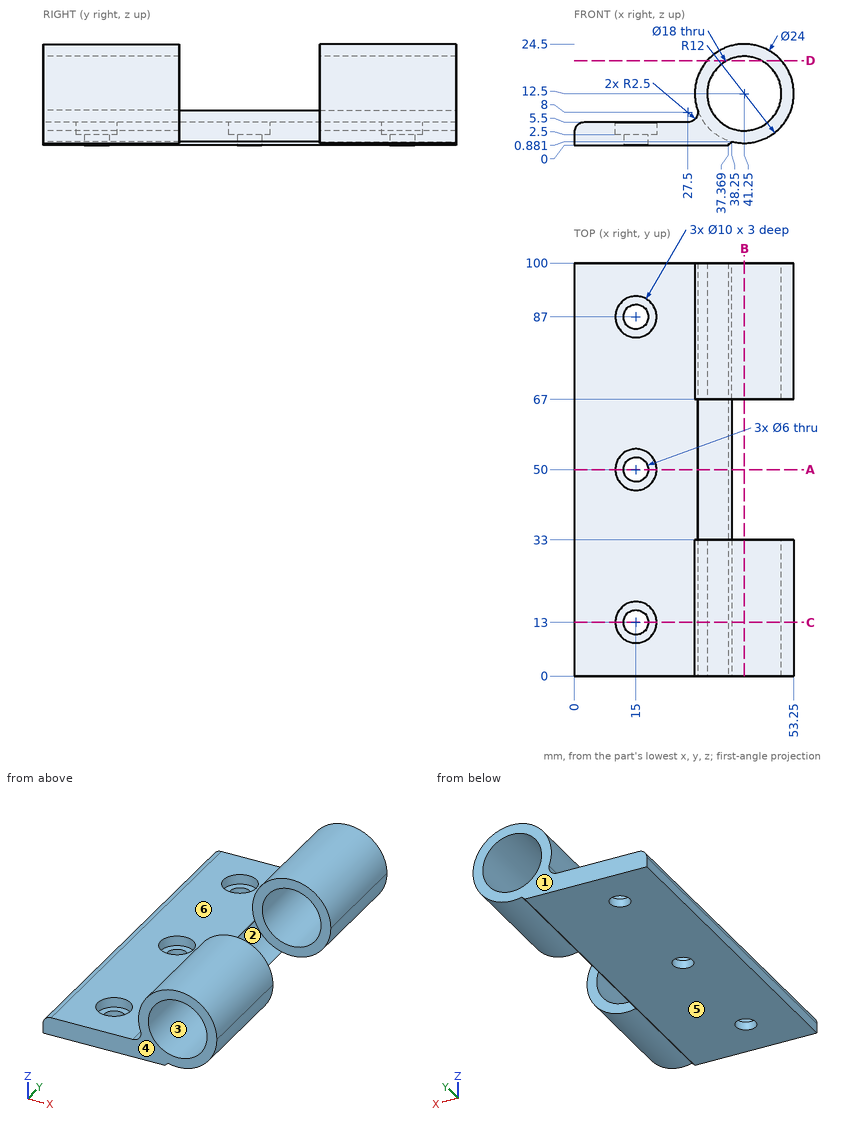
Geometry check sheet. Reference: drawing and pictorial views, mm from the part's lowest x, y, z. A direction names the side the tool comes from. Give positions to 0.01 mm unless a question says otherwise; leave off trailing zeros. Loops run counter-clockwise (first coordinate to the right, second up) from the corner with the lowest first, then second, coordinate; pieces in that order, holes last. Notation, with made-up numbers: (72, 53.25) - (102, 53.25) arc R33 cw to (102, 83.25) - close; hole circle Ø1 at (-5.5, -19.5). An arc over 180 degrees is marked (long way). Use CSV: the item, a comma, the result in double quotes. Start each with the question number.
Q1. Access from +Z, -Z, +X, -X, +Y, -Y to the whole of each face (thin tool, end or side, straight path). Record for the marked faces 1 and 2.
Q2. Go/stop test with flat-tipped pins: pin 1 Ø8 at (y, z) = (89, 4) entering from +X; pin 2 Ø1 at (x, y) = (8, 30) entering from -Z; pin 3 Ø9.5 at (x, y) = (15, 87) entering from +Z; pin 4 Ø11 at (x, y) = (13, 48) entering from +Z. Record where each tip stops, or that it passes through.
Q3. Section check A-A, the plane y = 50. Record the cut outline in (x, z), and give its area (3 significant figures).
Q4. Release check for a two-part mould opening along Z. For the marked faces 3, 4, 5 and 6 record: +Z half, -Z half, draft (parallel to the pull), parting line (faces both ways), or undercut.
Q5. Section check C-C, the plane y = 13. Record the cut outline in (x, z), and give its area (3 significant figures).
Q6. Section check B-B, the plane x = 41.25. Record the cut outline in (y, z).
Q7. Scan lines: probe 1 along Y at (x, z) = (15, 1.65); probe 2 along Z at (x, y) = (41.25, 19.5); probe 3 along Y at (x, z) = (34, 3). Record each from-to range of solid material in increasing order. Write a range as from..to.
Q8. Section check D-D, the plane z = 20.5. Record the cut outline in (x, y).
Findings below:
1,face 1,"+Z, -Z, +X, -X, +Y"
1,face 2,"+Z, +X"
2,pin 1,"stops at x = 52.37"
2,pin 2,"stops at z = 0"
2,pin 3,"stops at z = 2.5"
2,pin 4,"stops at z = 5.5"
3,outline,"(0, 0) - (12, 0) - (12, 2.5) - (10, 2.5) - (10, 5.5) - (2.5, 5.5) arc R2.5 ccw to (0, 3) - close; (18, 0) - (37.37, 0) - (38.25, 0.88) arc R12 cw to (29.96, 8.42) arc R2.5 cw to (27.5, 5.5) - (20, 5.5) - (20, 2.5) - (18, 2.5) - close"
3,area,"147 mm^2"
4,face 3,"undercut"
4,face 4,"draft"
4,face 5,"-Z half"
4,face 6,"+Z half"
5,outline,"(0, 0) - (12, 0) - (12, 2.5) - (10, 2.5) - (10, 5.5) - (2.5, 5.5) arc R2.5 ccw to (0, 3) - close; (18, 0) - (37.37, 0) - (38.25, 0.88) arc R12 ccw (long way) to (29.96, 8.42) arc R2.5 cw to (27.5, 5.5) - (20, 5.5) - (20, 2.5) - (18, 2.5) - close; hole circle Ø18 at (41.25, 12.5)"
5,area,"345 mm^2"
6,outline,"(0, 0.5) - (33, 0.5) - (33, 3.5) - (0, 3.5) - close; (0, 21.5) - (33, 21.5) - (33, 24.5) - (0, 24.5) - close; (67, 0.5) - (100, 0.5) - (100, 3.5) - (67, 3.5) - close; (67, 21.5) - (100, 21.5) - (100, 24.5) - (67, 24.5) - close"
7,probe 1,"y = 0..10, 16..47, 53..84, 90..100"
7,probe 2,"z = 0.5..3.5, 21.5..24.5"
7,probe 3,"y = 0..33, 67..100"
8,outline,"(32.31, 0) - (37.13, 0) - (37.13, 33) - (32.31, 33) - close; (32.31, 67) - (37.13, 67) - (37.13, 100) - (32.31, 100) - close; (45.37, 0) - (50.19, 0) - (50.19, 33) - (45.37, 33) - close; (45.37, 67) - (50.19, 67) - (50.19, 100) - (45.37, 100) - close"
